```python
from build123d import *

# Parameters (mm, degrees)
F1_DEPTH    = 10
F3_D        = 6.6
F6_D        = 5
F6_DEPTH    = 22
F6_TIP      = 1.5021515476
F7_R        = 1
F8_C1_SIZE  = 0.5
F8_C2_SIZE  = 0.5
F8_C3_SIZE  = 0.5
F8_C4_SIZE  = 0.5
F8_C5_SIZE  = 0.5
F8_C6_SIZE  = 0.5
F8_C7_SIZE  = 0.5
F8_C8_SIZE  = 0.5
F8_C9_SIZE  = 0.5
F8_C10_SIZE = 0.5
F8_C11_SIZE = 0.5
F8_C12_SIZE = 0.5


with BuildPart() as f1:
    # F0 (on Front) → F1 (new body, symmetric)
    with BuildSketch(Plane.XZ):
        with BuildLine():
            Line((15, 51), (0.5, 51))
            Line((0.5, 51), (0.5, 40.9874921777))
            ThreePointArc((0.5, 40.9874921777), (9.9968725554, 30.7499217894), (0, 21))
            Line((0, 21), (0, 0))
            Line((0, 0), (30, 0))
            Line((30, 0), (30, 10))
            Line((30, 10), (15, 10))
            Line((15, 10), (15, 51))
        make_face()
    extrude(amount=F1_DEPTH, both=True)

    # F3 (through all)
    with Locations(Plane(origin=(0, 0, 0), x_dir=(1, 0, 0), z_dir=(0, 0, -1))):
        with Locations((22.5, 0)):
            Hole(F3_D / 2)

    # F4: F1 across plane


with BuildPart() as f1_1:
    add(f1.part)
    add(f1.part.mirror(Plane.YZ))

    # F6
    with Locations(Plane.YZ.offset(15)):
        with Locations((0, 46)):
            Hole(F6_D / 2, depth=F6_DEPTH)
            with Locations((0, 0, -(F6_DEPTH + F6_TIP / 2))):  # 118° drill point
                Cone(0, F6_D / 2, F6_TIP, mode=Mode.SUBTRACT)

    # F7
    f7_edges = [f1_1.edges().sort_by_distance(p)[0] for p in [
        (15, 0, 10),
        (-15, 0, 10),
        (-30, 0, 10),
        (30, 0, 10),
        (15, 0, 51),
        (-15, 0, 51),
    ]]
    fillet(f7_edges, radius=F7_R)

    # F8: chamfer of 0.5 on 36 edges, made by hand

    # F8_c1
    f8_c1_edges = [f1_1.edges().sort_by_distance(p)[0] for p in [
        (30, 10, 4.5),
        (29.7071067812, 10, 9.7071067812),
        (22.5, 10, 10),
        (15.2928932188, 10, 10.2928932188),
        (15, 10, 30.5),
        (14.7071067812, 10, 50.7071067812),
        (7.25, 10, 51),
    ]]
    chamfer(f8_c1_edges, length=F8_C1_SIZE)

    # F8_c2
    f8_c2_edges = [f1_1.edges().sort_by_distance(p)[0] for p in [
        (-0.25, 10, 0),
    ]]
    chamfer(f8_c2_edges, length=F8_C2_SIZE)

    # F8_c3
    f8_c3_edges = [f1_1.edges().sort_by_distance(p)[0] for p in [
        (-30, 10, 4.75),
        (-29.7071067812, 10, 9.7071067812),
        (-22.5, 10, 10),
        (-15.2928932188, 10, 10.2928932188),
        (-15, 10, 30.5),
        (-14.7071067812, 10, 50.7071067812),
        (-7.25, 10, 51),
    ]]
    chamfer(f8_c3_edges, length=F8_C3_SIZE)

    # F8_c4
    f8_c4_edges = [f1_1.edges().sort_by_distance(p)[0] for p in [
        (0.5, 10, 45.7437460889),
    ]]
    chamfer(f8_c4_edges, length=F8_C4_SIZE)

    # F8_c5
    f8_c5_edges = [f1_1.edges().sort_by_distance(p)[0] for p in [
        (-0.2507065513, 10, 21.0031431827),
    ]]
    chamfer(f8_c5_edges, length=F8_C5_SIZE)

    # F8_c6
    f8_c6_edges = [f1_1.edges().sort_by_distance(p)[0] for p in [
        (-0.5, 10, 45.9940442409),
    ]]
    chamfer(f8_c6_edges, length=F8_C6_SIZE)

    # F8_c7
    f8_c7_edges = [f1_1.edges().sort_by_distance(p)[0] for p in [
        (30, -10, 4.5),
        (29.7071067812, -10, 9.7071067812),
        (22.5, -10, 10),
        (15.2928932188, -10, 10.2928932188),
        (15, -10, 30.5),
        (14.7071067812, -10, 50.7071067812),
        (7.25, -10, 51),
    ]]
    chamfer(f8_c7_edges, length=F8_C7_SIZE)

    # F8_c8
    f8_c8_edges = [f1_1.edges().sort_by_distance(p)[0] for p in [
        (-0.25, -10, 0),
    ]]
    chamfer(f8_c8_edges, length=F8_C8_SIZE)

    # F8_c9
    f8_c9_edges = [f1_1.edges().sort_by_distance(p)[0] for p in [
        (-30, -10, 4.75),
        (-29.7071067812, -10, 9.7071067812),
        (-22.5, -10, 10),
        (-15.2928932188, -10, 10.2928932188),
        (-15, -10, 30.5),
        (-14.7071067812, -10, 50.7071067812),
        (-7.25, -10, 51),
    ]]
    chamfer(f8_c9_edges, length=F8_C9_SIZE)

    # F8_c10
    f8_c10_edges = [f1_1.edges().sort_by_distance(p)[0] for p in [
        (0.5, -10, 45.7437460889),
    ]]
    chamfer(f8_c10_edges, length=F8_C10_SIZE)

    # F8_c11
    f8_c11_edges = [f1_1.edges().sort_by_distance(p)[0] for p in [
        (-0.2507065513, -10, 21.0031431827),
    ]]
    chamfer(f8_c11_edges, length=F8_C11_SIZE)

    # F8_c12
    f8_c12_edges = [f1_1.edges().sort_by_distance(p)[0] for p in [
        (-0.5, -10, 45.9940442409),
    ]]
    chamfer(f8_c12_edges, length=F8_C12_SIZE)


solid = f1_1.part
```
Geometry: final body of the model. Coordinates: model frame, mm. A direction names the side the tool comes from. Coordinates: 2 decimals unless noted, no trailing zeros. Loops run counter-clockwise (first coordinate to the right, second up) from the corner with the lowest first, then second, coordinate; pieces in that order, holes last. Notation, with made-up numbers: M 78.5,-3 L 92.5,-3 A12 ccw 92.5,12 Z; hole C -18.75,24.5 d4. An arc over 180 degrees is marked long. Put each result on its own line as item: value.
(1) Cut plane D-D on z = 7. Return the cut outline in (x, y), then the cut area to 3 significant figures.
Answer sheet:
outline: M -30,-9.5 L -29.5,-10 L 29.5,-10 L 30,-9.5 L 30,9.5 L 29.5,10 L -29.5,10 L -30,9.5 Z; hole C -22.5,0 d6.6; hole C 22.5,0 d6.6
area: 1,130 mm^2
(2) Draft query along X for faces 1 (the face through (7, 0, 51)), 2 (the face through (19.45, 1.26, 5.07)), 3 (the face through (-30, 0, 4)), 4 (the face through (0.5, -2, 48)). Return one class per face: pulls with the +X half, pulls with the -X half, needs draft (parallel to the pull), parting line crosses it, or undercut.
Answer sheet:
face 1: needs draft
face 2: undercut
face 3: pulls with the -X half
face 4: undercut
(3) Cut plane C-C on y = 5.5. Return the cut outline in (x, z).
Answer sheet:
outline: M -30,0 L 30,0 L 30,9 A1 ccw 29,10 L 16,10 A1 cw 15,11 L 15,50 A1 ccw 14,51 L 0.5,51 L 0.5,40.99 A10 cw long -0.5,40.99 L -0.5,51 L -14,51 A1 ccw -15,50 L -15,11 A1 cw -16,10 L -29,10 A1 ccw -30,9 Z
(4) Cut plane A-A on x = 22.5. Return the cut outline in (y, z).
Answer sheet:
outline: M -10,0.5 L -9.5,0 L -3.3,0 L -3.3,10 L -9.5,10 L -10,9.5 Z; M 3.3,0 L 9.5,0 L 10,0.5 L 10,9.5 L 9.5,10 L 3.3,10 Z
(5) Material intervals for probe 1 along Y at (x, z) = (-22.5, 4.25); probe 2 along Z at (x, y) = (-18, -6.25); probe 3 along X at (y, z) = (-2.5, 23), sorted ascending.
Answer sheet:
probe 1: y = -10 to -3.3, 3.3 to 10
probe 2: z = 0 to 10
probe 3: x = -15 to -6, 6 to 15
(6) Access query for faces 5 (the face through (-25.5, -2.2, 10)), 6 (the face through (-3.8, 0.54, 43.56)), 7 (the face through (25.5, -2.2, 10)). Directions: +Z, -Z, +X, -X, +Y, -Y. A direction counts if a zero-diameter tool reaches every point of the face in a straight line with its end or side. Return the directions, or none.
Answer sheet:
face 5: +Z, -X, +Y, -Y
face 6: +X
face 7: +Z, +X, +Y, -Y
(7) Cut plane B-B on z = 19. Return the cut outline in (x, y).
Answer sheet:
outline: M -15,-9.5 L -14.5,-10 L 14.5,-10 L 15,-9.5 L 15,9.5 L 14.5,10 L -14.5,10 L -15,9.5 Z
(8) First-contact query: pin 1 (11 mm diameter, centred on y = 0.5, z = 43.5, fed in from -X); pin 2 (3 mm diameter, centred on y = -5.5, z = 32, fed in from +X); pin 3 (10.5 mm diameter, centred on x = -22, y = 4.5, fed in from +Z). Flat tips, straight axial feed; report the tip coordinate or a pass-through.
Answer sheet:
pin 1: stops at x = -15
pin 2: stops at x = 15
pin 3: stops at z = 10
